Could you check a few things on this drawing? It's one solid part, dimensions in mm from its lowest x, y, z. A direction names the side the tool comes from. Round coordinates to 2 decimals unless told otherwise and drop trailing zeros. Order: outer loops, then holes, each group sorted by start corner. A loop starts at its lowest first (then second) coordinate and runs counter-clockwise, first axis right, second up. Notation, with made-up numbers: (56, 77) -> (108, 77) arc R13 cw to (108, 89) -> close; hole circle Ø1 at (46.25, 89.25). An arc over 180 degrees is marked (long way). Use a Markdown table: item, result. Add a question column.
(1) I want a section at A-A, the plane z = 15. Please give me the cut outline in (x, y).
(2) I'm going to push flat-ended pins straight in: P1, Ø3, axis at x = 3, y = 10.5, coming from the -Z side; P2, Ø2, axis at y = 17, z = 19.5, coming from the +X side; P3, Ø4, axis at x = 26.5, z = 17.5, coming from the +Y side; P4, Ø4, axis at x = 63.5, z = 40, coming from the -Y side. Where does each tip first touch, or does it pass through?
(3) On a 3-axis mill with a long thin cutter (end or side, diameter ignored), from which of +Z, -Z, +X, -X, +Y, -Y can I reach the whole of each face in a straight line? I mean the marked faces 1 and 2. Say none if no direction works.
(4) If I drill on probe 1 along X at (y, z) = (18.75, 15); probe 2 along Z at (x, y) = (22, 19); probe 3 along X at (y, z) = (18.5, 38), over which ranges is the centre line in solid material (lowest first)?
(5) I want a section at D-D, the plane y = 18.25. Please give me the cut outline in (x, z), then the cut area to 3 significant figures.
(6) I want a section at C-C, the plane x = 22. Please give me the cut outline in (y, z), then the cut area to 3 significant figures.
(7) I want a section at B-B, the plane y = 2. Please give me the cut outline in (x, z), then the cut area to 3 significant figures.
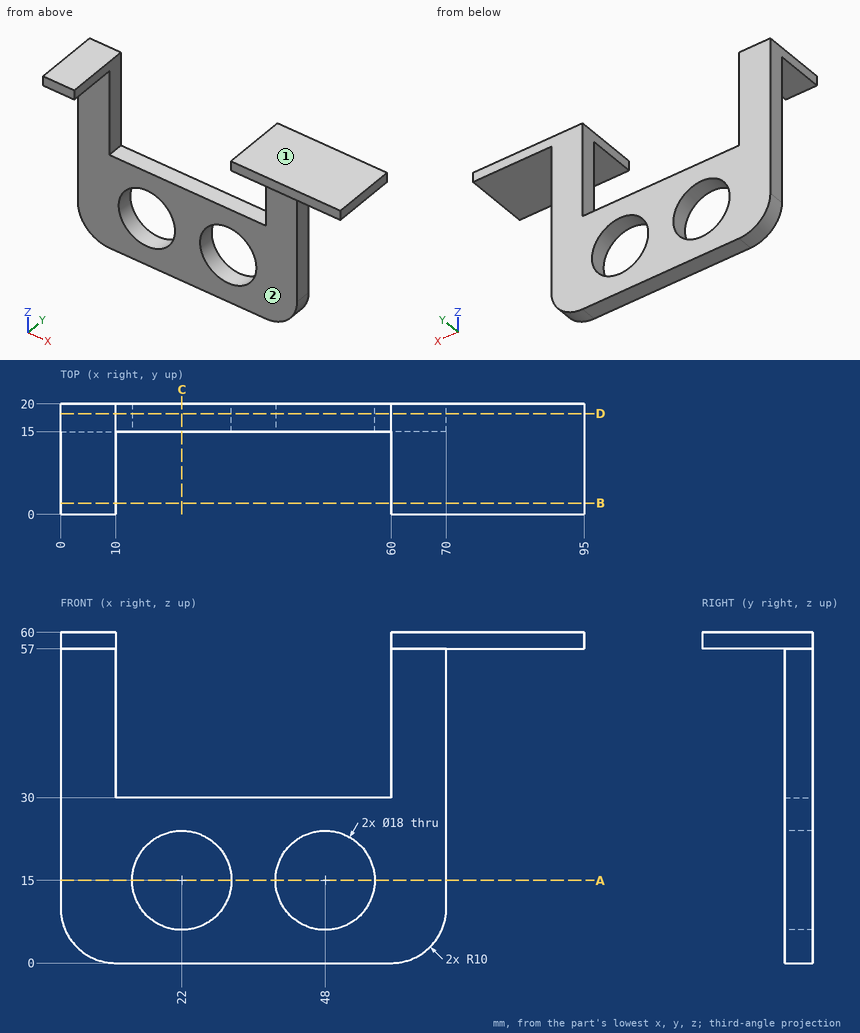
Taken from the geometry:
| question | item | result |
|---|---|---|
| 1 | outline | (0, 15) -> (13, 15) -> (13, 20) -> (0, 20) -> close; (31, 15) -> (39, 15) -> (39, 20) -> (31, 20) -> close; (57, 15) -> (70, 15) -> (70, 20) -> (57, 20) -> close |
| 2 | P1 | stops at z = 57 |
| 2 | P2 | stops at x = 70 |
| 2 | P3 | passes through |
| 2 | P4 | stops at y = 15 |
| 3 | face 1 | +Z, +X, -X, +Y, -Y |
| 3 | face 2 | -Z, +X, -X, -Y |
| 4 | probe 1 | x = 0 to 13, 31 to 39, 57 to 70 |
| 4 | probe 2 | z = 0 to 6, 24 to 30 |
| 4 | probe 3 | x = 0 to 10, 60 to 70 |
| 5 | outline | (0, 10) arc R10 ccw to (10, 0) -> (60, 0) arc R10 ccw to (70, 10) -> (70, 57) -> (95, 57) -> (95, 60) -> (60, 60) -> (60, 30) -> (10, 30) -> (10, 60) -> (0, 60) -> close; hole circle Ø18 at (22, 15); hole circle Ø18 at (48, 15) |
| 5 | area | 2,220 mm2 |
| 6 | outline | (15, 0) -> (20, 0) -> (20, 6) -> (15, 6) -> close; (15, 24) -> (20, 24) -> (20, 30) -> (15, 30) -> close |
| 6 | area | 60.0 mm2 |
| 7 | outline | (0, 57) -> (10, 57) -> (10, 60) -> (0, 60) -> close; (60, 57) -> (95, 57) -> (95, 60) -> (60, 60) -> close |
| 7 | area | 135 mm2 |
